```python
from build123d import *

# Parameters (mm, degrees)
SKETCH5_W                 = 11.25
SKETCH5_H                 = 8.5
EXTRUDE4_DEPTH            = 2.5
SKETCH19_W                = 1.5
SKETCH19_H                = 8.5
EXTRUDE12_DEPTH           = 1.5
SKETCH21_W                = 9
SKETCH21_H                = 7
EXTRUDE13_DEPTH           = 3.5
SKETCH22_W                = 4
SKETCH22_H                = 2.5
EXTRUDE14_DEPTH           = 3.75
EXTRUDE15_DEPTH           = 0.75
F_0_80_TAPPED_HOLE1_D     = 1.19126
F_0_80_TAPPED_HOLE1_DEPTH = 79.01
F_0_80_TAPPED_HOLE1_TIP   = 0.357890611
FILLET4_R                 = 1


with BuildPart() as part:
    # Sketch5 → Extrude4 (new body)
    with BuildSketch(Plane(origin=(0, 0, 0), x_dir=(1, 0, 0), z_dir=(0, 1, 0))):
        Rectangle(SKETCH5_W, SKETCH5_H)
    extrude(amount=EXTRUDE4_DEPTH)

    # Sketch19 → Extrude12 (cut)
    with BuildSketch(Plane(origin=(0, 2.5, 0), x_dir=(-1, 0, 0), z_dir=(0, 1, 0))):
        with Locations((4.875, 0)):
            Rectangle(SKETCH19_W, SKETCH19_H)
    extrude(amount=-EXTRUDE12_DEPTH, mode=Mode.SUBTRACT)

    # Sketch21 → Extrude13 (cut, through all)
    with BuildSketch(Plane(origin=(0, 2.5, 0), x_dir=(-1, 0, 0), z_dir=(0, 1, 0))):
        with Locations((-0.375, 0)):
            Rectangle(SKETCH21_W, SKETCH21_H)
    extrude(amount=-EXTRUDE13_DEPTH, mode=Mode.SUBTRACT)

    # Sketch22 → Extrude14 (add)
    with BuildSketch(Plane.XY.offset(4.25)):
        with Locations((-0.875, 1.25)):
            Rectangle(SKETCH22_W, SKETCH22_H)
    extrude(amount=EXTRUDE14_DEPTH)

    # Sketch24 → Extrude15 (add)
    with BuildSketch(Plane(origin=(0, 2.5, 0), x_dir=(1, 0, 0), z_dir=(0, 1, 0))):
        Polygon((-4.125, 3.85), (-4.125, 3.5), (4.875, 3.5), (4.875, -3.5), (-4.125, -3.5), (-4.125, -3.85), (5.225, -3.85), (5.225, 3.85), align=None)
    extrude(amount=EXTRUDE15_DEPTH)

    # #0-80 Tapped Hole1
    with Locations(Plane(origin=(-0.875, 2.5, 6), x_dir=(0, 0, 1), z_dir=(0, 1, 0))):
        with Locations((0, 0)):
            Hole(F_0_80_TAPPED_HOLE1_D / 2, depth=F_0_80_TAPPED_HOLE1_DEPTH)
            with Locations((0, 0, -(F_0_80_TAPPED_HOLE1_DEPTH + F_0_80_TAPPED_HOLE1_TIP / 2))):  # 118° drill point
                Cone(0, F_0_80_TAPPED_HOLE1_D / 2, F_0_80_TAPPED_HOLE1_TIP, mode=Mode.SUBTRACT)

    # Fillet4
    fillet4_edges = [part.edges().sort_by_distance(p)[0] for p in [
        (5.625, 1.25, -4.25),
        (5.225, 2.875, -3.85),
        (5.625, 1.25, 4.25),
        (5.225, 2.875, 3.85),
        (4.875, 1.625, 3.5),
        (4.875, 1.625, -3.5),
        (-4.125, 0.5, 3.5),
        (-4.125, 0.5, -3.5),
        (-5.625, 0.5, -4.25),
        (-5.625, 0.5, 4.25),
        (-2.875, 1.25, 4.25),
        (-2.875, 1.25, 8),
        (1.125, 1.25, 8),
        (1.125, 1.25, 4.25),
    ]]
    fillet(fillet4_edges, radius=FILLET4_R)


solid = part.part
```
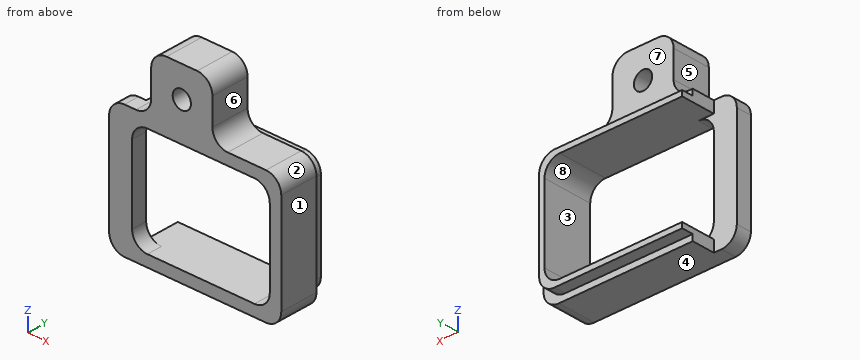
The listing builds one solid part. Answer for the finished solid, in the listing's coordinates (mm). Face numbers are marked on the shaded views. A direction names the side the tool comes from. Coordinates: 2 decimals unless noted, no trailing zeros. Loops run counter-clockwise (first coordinate to the right, second up) from the corner with the lowest first, then second, coordinate; pieces in that order, holes last. Notation, with made-up numbers: (77.25, 66) -> (121.25, 66) arc R16 cw to (121.25, 72) -> close; hole circle Ø9 at (75, -11.5). An arc over 180 degrees is marked (long way). Return JSON: item names as keys, results as strings. Group by question number.
(1) Given pin 1 Ø1 at (y, z) = (2, 2) entering from -X (3 decimals); pin 2 Ø0.5 at (y, z) = (1, 6) entering from -X (3 decimals); pin 3 Ø0.8 at (x, y) = (0, 3) entering from -Z, each flat-ended and moving along its own axis, determine where each tip first touches the part or whether it passes through.
(2) A cutting plane is placed at A-A on z = 0.5. Write down the section's boundary in (x, y) (3 decimals), and give its area (3 significant figures).
(3) Find the intervals of material crossed by probe 1 along X at (y, z) = (1.1, 6) (3 decimals); probe 2 along Z at (x, y) = (2, 3.15); probe 3 along X at (y, z) = (0.3, 0.75) (3 decimals), in increasing order. Write a range as from..to.
(4) A cutting plane is placed at C-C on y = 2.25. Write down the section's boundary in (x, z) (3 decimals).
(5) A cutting plane is placed at D-D on z = 6. Write down the section's boundary in (x, y) (3 decimals), and give its area (3 significant figures).
(6) Which of the six approach directions +Z, -Z, +X, -X, +Y, -Y give full straight-line access (tool end or side, diameter ignored) to the marked faces 4, 5, 6, 7 and 8?
(7) Determine the mould class of the marked faces 1, 2 and 3 for opening direction Z: released by +Z, released by -Z, zero draft, split by the parting line, or undercut.
(8) A cutting plane is placed at B-B on y = 0.2. Write down the section's boundary in (x, z) (3 decimals).
The answers:
{
 "1": {"pin 1": "stops at x = 4.875", "pin 2": "stops at x = -2.875", "pin 3": "stops at z = -3.85"},
 "2": {"outline": "(-5.625, 0) -> (-4.125, 0) -> (-4.125, 1) -> (-5.625, 1) -> close; (4.875, 0) -> (5.625, 0) -> (5.625, 2.5) -> (5.225, 2.5) -> (5.225, 3.25) -> (4.875, 3.25) -> close", "area": "3.64 mm^2"},
 "3": {"probe 1": "x = -2.875..-1.471, -0.279..1.125", "probe 2": "z = -3.85..-3.5, 3.5..3.85", "probe 3": "x = -5.625..-4.125, 4.875..5.625"},
 "4": {"outline": "(-4.125, -4.25) -> (4.625, -4.25) arc R1 ccw to (5.625, -3.25) -> (5.625, 3.25) arc R1 ccw to (4.625, 4.25) -> (2.125, 4.25) arc R1 cw to (1.125, 5.25) -> (1.125, 7) arc R1 ccw to (0.125, 8) -> (-1.875, 8) arc R1 ccw to (-2.875, 7) -> (-2.875, 5.25) arc R1 cw to (-3.875, 4.25) -> (-4.125, 4.25) -> (-4.125, 3.5) -> (3.875, 3.5) arc R1 cw to (4.875, 2.5) -> (4.875, -2.5) arc R1 cw to (3.875, -3.5) -> (-4.125, -3.5) -> close; hole circle Ø1.191 at (-0.875, 6)"},
 "5": {"outline": "(-2.875, 0) -> (-1.471, 0) -> (-1.471, 2.5) -> (-2.875, 2.5) -> close; (-0.279, 0) -> (1.125, 0) -> (1.125, 2.5) -> (-0.279, 2.5) -> close", "area": "7.02 mm^2"},
 "6": {"face 4": "-Z, +X, -X, +Y, -Y", "face 5": "+Z, -X, +Y, -Y", "face 6": "+Z, +X, +Y, -Y", "face 7": "+X, +Y", "face 8": "+Y, -Y"},
 "7": {"face 1": "zero draft", "face 2": "released by +Z", "face 3": "undercut"},
 "8": {"outline": "(-5.625, -3.25) arc R1 ccw to (-4.625, -4.25) -> (4.625, -4.25) arc R1 ccw to (5.625, -3.25) -> (5.625, 3.25) arc R1 ccw to (4.625, 4.25) -> (2.125, 4.25) arc R1 cw to (1.125, 5.25) -> (1.125, 7) arc R1 ccw to (0.125, 8) -> (-1.875, 8) arc R1 ccw to (-2.875, 7) -> (-2.875, 5.25) arc R1 cw to (-3.875, 4.25) -> (-4.625, 4.25) arc R1 ccw to (-5.625, 3.25) -> close; hole (-4.125, -2.5) arc R1 ccw to (-3.125, -3.5) -> (3.875, -3.5) arc R1 ccw to (4.875, -2.5) -> (4.875, 2.5) arc R1 ccw to (3.875, 3.5) -> (-3.125, 3.5) arc R1 ccw to (-4.125, 2.5) -> close; hole circle Ø1.191 at (-0.875, 6)"}
}
